```python
from build123d import *

# Parameters (mm, degrees)
SKETCH3_W          = 4.079746654
SKETCH3_H          = 4
CUT_EXTRUDE1_DEPTH = 51
CUT_EXTRUDE2_START = 11
CUT_EXTRUDE2_DEPTH = 1.7
CHAMFER1_SIZE      = 1
FILLET1_R          = 1


with BuildPart() as part:
    # Sketch2 → Revolve1 (revolve)
    with BuildSketch(Plane(origin=(0, 0, 0), x_dir=(1, 0, 0), z_dir=(0, 1, 0)), mode=Mode.PRIVATE) as revolve1_sk:
        Polygon((0, 0), (-9.25, 0), (-9.25, 72), (-9.5, 72), (-9.5, 87), (-13, 87), (-13, 109), (-11, 109), (-11, 153), (-9.5, 153), (-9.5, 168), (0, 168), align=None)
    revolve(revolve1_sk.sketch.rotate(Axis((0, 0, 0), (0, 0, -1)), 180), axis=Axis((0, 0, 0), (0, 0, -1)))

    # Sketch3 → Cut-Extrude1 (cut)
    with BuildSketch(Plane.XY):
        with Locations((9.589873327, 0)):
            Rectangle(SKETCH3_W, SKETCH3_H)
    extrude(amount=-CUT_EXTRUDE1_DEPTH, mode=Mode.SUBTRACT)

    # Sketch4 → Cut-Extrude2 (cut)
    with BuildSketch(Plane(origin=(0, 0, 0), x_dir=(0, 0, -1), z_dir=(1, 0, 0)).offset(CUT_EXTRUDE2_START)):
        with BuildLine():
            Line((117, 2), (131, 2))
            ThreePointArc((131, 2), (133, 0), (131, -2))
            Line((131, -2), (117, -2))
            ThreePointArc((117, -2), (115, 0), (117, 2))
        make_face()
    extrude(amount=-CUT_EXTRUDE2_DEPTH, mode=Mode.SUBTRACT)

    # Chamfer1
    chamfer1_edges = [part.edges().sort_by_distance(p)[0] for p in [
        (-9.25, 0, 0),
        (-9.5, 0, -168),
    ]]
    chamfer(chamfer1_edges, length=CHAMFER1_SIZE)

    # Fillet1
    fillet1_edges = [part.edges().sort_by_distance(p)[0] for p in [
        (7.55, 0, -51),
    ]]
    fillet(fillet1_edges, radius=FILLET1_R)


solid = part.part
```
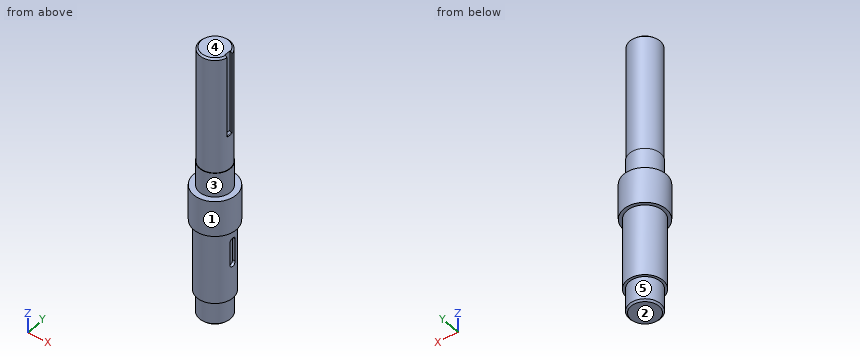
Work out the finished part from the listing and answer in its coordinate system (mm). Face numbers are marked on the shaded views. A direction names the side the tool comes from. Give positions to 0.01 mm unless a question says otherwise; leave off trailing zeros. Loops run counter-clockwise (first coordinate to the right, second up) from the corner with the lowest first, then second, coordinate; pieces in that order, holes last. Notation, with made-up numbers: M -5,23.5 L 26,23.5 A22 ccw 26,37.5 Z; hole C -31,-2 d4. An arc over 180 degrees is marked long. One line per item, written item: value. Start each with the question number.
1. Find section D-D (z = -83.5). Give the vertices of the cut face in (x, y), and give its area (3 significant figures).
2. Which of the six approach directions +Z, -Z, +X, -X, +Y, -Y give full straight-line access (tool end or side, diameter ignored) to the marked faces 3, 4 and 5?
3. Each of these flat-tipped pins is pushed along its axis until it touches: P1, Ø3, axis at x = -9.5, z = -104, coming from the +Y side; P2, Ø6, axis at x = 8, y = 9.5, coming from the -Z side; P3, Ø8, axis at x = 3.5, z = -136.5, coming from the +Y side. Where does it stop, or does it pass through?
4. Find section C-C (z = -55.5). Give the vertices of the cut face in (x, y), and give its area (3 significant figures).
5. Find section A-A (x = 0). Give the vertices of the cut face in (y, z), and give its area (3 significant figures).
6. Determine the mould class of the marked faces 1 and 2 for opening direction Y: released by +Y, released by -Y, zero draft, split by the parting line, or undercut.
7. Find the intervals of material crossed by probe 1 along Z at (x, y) = (-10.25, -7.25); probe 2 along Z at (x, y) = (-9.5, -3.75); probe 3 along Y at (x, z) = (4.75, -140), in increasing order.
Reported:
1. outline: C 0,0 d19
1. area: 284 mm²
2. face 3: +Z
2. face 4: +Z, +X, -X, +Y, -Y
2. face 5: -Z
3. P1: stops at y = 10.25
3. P2: stops at z = -167.08
3. P3: stops at y = 11
4. outline: C 0,0 d18.5
4. area: 269 mm²
5. outline: M -13,-109 L -11,-109 L -11,-153 L -9.5,-153 L -9.5,-167 L -8.5,-168 L 8.5,-168 L 9.5,-167 L 9.5,-153 L 11,-153 L 11,-109 L 13,-109 L 13,-87 L 9.5,-87 L 9.5,-72 L 9.25,-72 L 9.25,-1 L 8.25,0 L -8.25,0 L -9.25,-1 L -9.25,-72 L -9.5,-72 L -9.5,-87 L -13,-87 Z
5. area: 3,440 mm²
6. face 1: split by the parting line
6. face 2: zero draft
7. probe 1: z = -109 to -87
7. probe 2: z = -153 to -87
7. probe 3: y = -9.92 to 9.92
